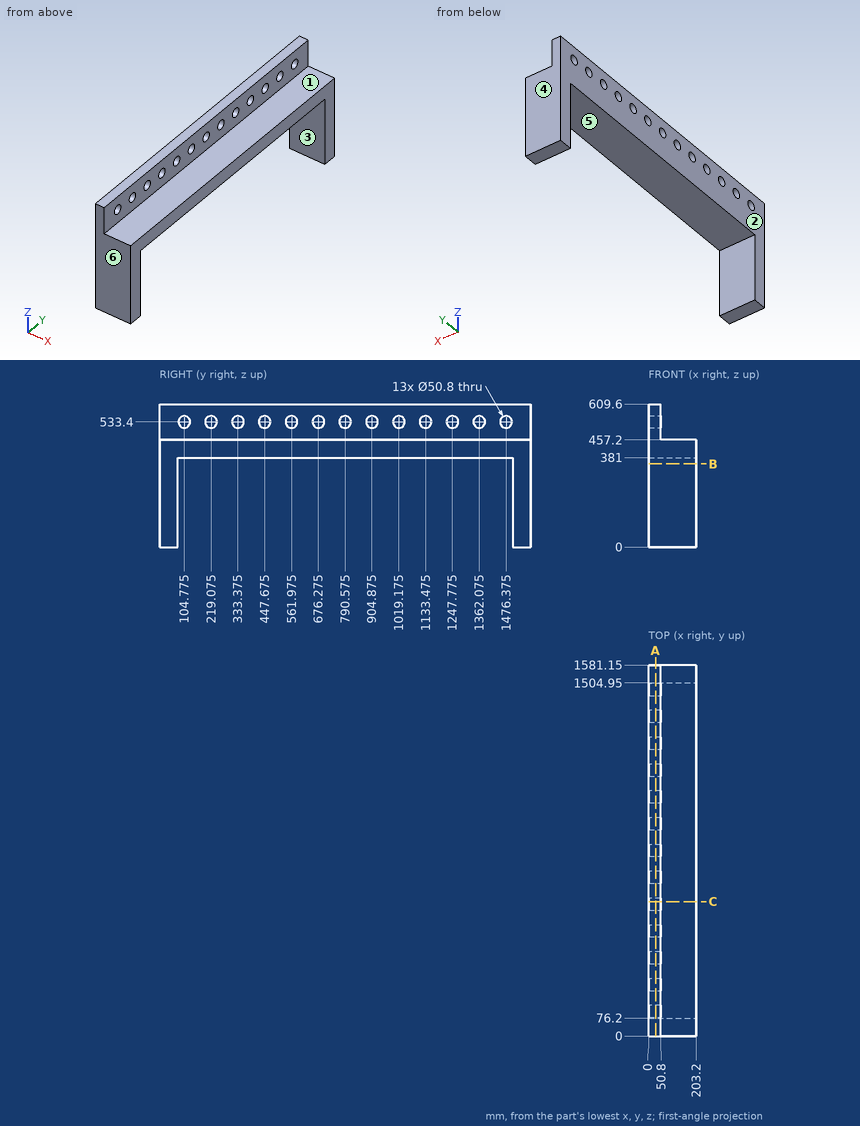
Design review of the part shown in the three views and the two pictorial views. Dimensions are in mm from the part's minimum x, y and z. A direction names the side the tool comes from. Round coordinates to 2 decimals unless told otherwise and drop trailing zeros. Write each loop counter-clockwise with the first axis right and the second up, starting at its lowest first coordinate (ties: lowest second). Pieces come first, ordered by that corner, then holes. Notation, with made-up numbers: (33, 8.5) -> (82, 8.5) arc R18 ccw to (82, 28.5) -> close; hole circle Ø3 at (81, 16.5). An arc over 180 degrees is marked (long way). Answer as a JSON object with one key per item and string values.
1. We need section A-A on x = 30. State how many separate pieces and enclosed holes the cut face has, and give its area (3 significant figures).
Results found:
{"separate pieces": "1", "enclosed holes": "13", "area": "393,000 mm^2"}
2. We need section B-B on z = 354. State the section outline as (x, y) points, and give its area (3 significant figures).
Results found:
{"outline": "(0, 0) -> (203.2, 0) -> (203.2, 76.2) -> (0, 76.2) -> close; (0, 1504.95) -> (203.2, 1504.95) -> (203.2, 1581.15) -> (0, 1581.15) -> close", "area": "31,000 mm^2"}
3. We need section C-C on y = 572.5. State the section outline as (x, z) points, and give its area (3 significant figures).
Results found:
{"outline": "(0, 381) -> (203.2, 381) -> (203.2, 457.2) -> (50.8, 457.2) -> (50.8, 510.28) -> (0, 510.28) -> close; (0, 556.52) -> (50.8, 556.52) -> (50.8, 609.6) -> (0, 609.6) -> close", "area": "20,900 mm^2"}
4. Clearance check with flat-ended pins moving along their axes: pin 1 (5 mm diameter, centred on x = 131.5, z = 187.5, fed in from -Y); pin 2 (2 mm diameter, centred on x = 131, y = 1202, fed in from +Z). State where each tip first meets the part, or that it passes through.
Results found:
{"pin 1": "stops at y = 0", "pin 2": "stops at z = 457.2"}
5. Machinability: for the marked faces 1, 2 and 3, which of the approach directions +Z, -Z, +X, -X, +Y, -Y give a long, thin tool a straight path to every point of the face, cutting with its end or side? Answer none if there is none.
Results found:
{"face 1": "+Z, +X, +Y, -Y", "face 2": "+Z, -Z, -X, +Y, -Y", "face 3": "-Z, +X, -X"}
6. The part is to be moulded in two halves that separate along Y. For the marked faces 4, 5 and 6, say which applies: pulls with the +Y half, pulls with the -Y half, needs draft (parallel to the pull), parting line crosses it, or undercut.
Results found:
{"face 4": "pulls with the +Y half", "face 5": "undercut", "face 6": "pulls with the -Y half"}
7. To check wall thickness, follow line 1 along Y through (x, z) = (76, 378); line 2 along Z through (x, y) = (186, 1230.5); line 3 along X through (y, z) = (1172, 518). State the ranges of each line that lie inside material, in increasing order.
Results found:
{"line 1": "y = 0 to 76.2, 1504.95 to 1581.15", "line 2": "z = 381 to 457.2", "line 3": "x = 0 to 50.8"}
